Design review of the part built by this model. Coordinates are the model's own, in mm. A direction names the side the tool comes from. Round coordinates to 2 decimals unless told otherwise and drop trailing zeros. Order: outer loops, then holes, each group sorted by start corner. A loop starts at its lowest first (then second) coordinate and runs counter-clockwise, first axis right, second up. Notation, with made-up numbers: (66.5, 49.5) - (122.5, 49.5) arc R32 cw to (122.5, 82.5) - close; hole circle Ø8 at (77.5, 88.25). An arc over 180 degrees is marked (long way). Write item = value, one per line.
Autodesk Inventor part; units mm, degrees
ref_plane "YZ Plane" through (0, 0, 0) normal (1, 0, 0) x (0, 1, 0)
ref_plane "XZ Plane" through (0, 0, 0) normal (0, 1, 0) x (-1, 0, 0)
ref_plane "XY Plane" through (0, 0, 0) normal (0, 0, 1) x (1, 0, 0)
sketch "Esquisse1" plane through (0, 0, 0) normal (0, 1, 0) x (-1, 0, 0)
  line L0 (0, 0) -> (250, 0)
  line L1 (250, 0) -> (250, -32)
  line L2 (250, -32) -> (0, -32)
  line L3 (0, -32) -> (0, 0)
  circle A0 centre (2, -2) radius 1.5
  line L4 (250, -16) -> (0, -16) construction
  circle A1 centre (2, -30) radius 1.5
  circle A2 centre (51.1, -2) radius 1.5
  circle A3 centre (51.1, -30) radius 1.5
  circle A4 centre (100.2, -2) radius 1.5
  circle A5 centre (100.2, -30) radius 1.5
  circle A6 centre (149.3, -2) radius 1.5
  circle A7 centre (149.3, -30) radius 1.5
  circle A8 centre (198.4, -2) radius 1.5
  circle A9 centre (198.4, -30) radius 1.5
  circle A10 centre (247.5, -2) radius 1.5
  circle A11 centre (247.5, -30) radius 1.5
  dimension "d0" = 32
  dimension "d1" = 250
  dimension "d2" = 2
  dimension "d3" = 2
  dimension "d4" = 3
  dimension "d7" = 49.1
extrude "Extrusion1" add sketch "Esquisse1" along normal blind 1.6
sketch "Esquisse2" plane through (0, 1.6, 0) normal (0, 1, 0) x (1, 0, 0)
  circle A0 centre (-247.5, 30) radius 1.5 construction
  circle A1 centre (-247.5, 2) radius 1.5 construction
  circle A2 centre (-198.4, 30) radius 1.5 construction
  circle A3 centre (-198.4, 2) radius 1.5 construction
  circle A4 centre (-149.3, 30) radius 1.5 construction
  circle A5 centre (-149.3, 2) radius 1.5 construction
  circle A6 centre (-100.2, 30) radius 1.5 construction
  circle A7 centre (-100.2, 2) radius 1.5 construction
  circle A8 centre (-51.1, 30) radius 1.5 construction
  circle A9 centre (-51.1, 2) radius 1.5 construction
  circle A10 centre (-2, 30) radius 1.5 construction
  circle A11 centre (-2, 2) radius 1.5 construction
  line L0 (-250, 0) -> (0, 0) construction
  line L1 (0, 0) -> (0, 32) construction
  line L2 (0, 32) -> (-250, 32) construction
  line L3 (-250, 32) -> (-250, 0) construction
  line L4 (-246, 9.5) -> (-234, 9.5)
  line L5 (-234, 9.5) -> (-234, 21.5)
  line L6 (-234, 21.5) -> (-246, 21.5)
  line L7 (-246, 21.5) -> (-246, 9.5)
  dimension "d14" = 12
  dimension "d15" = 9.5
  dimension "d16" = 4
extrude "Extrusion2" add sketch "Esquisse2" along normal blind 7.7
sketch "Esquisse3" plane through (-246, 1.6, -21.5) normal (-1, 0, 0) x (0, 0, 1)
  circle A0 centre (4, 6) radius 1.1
  line L0 (-10.5, 0) -> (21.5, 0)
  line L1 (0, 0) -> (0, 7.7)
  line L2 (-10.5, -1.6) -> (21.5, -1.6)
  line L3 (5.5, -1.6) -> (5.5, 11.8569) construction
  dimension "d19" = 6
  dimension "d20" = 2.2
  dimension "d21" = 4
extrude "Extrusion3" add sketch "Esquisse3" along normal blind 7
sketch "Esquisse4" plane through (0, 1.6, 0) normal (0, 1, 0) x (1, 0, 0)
  line L0 (-246, 9.5) -> (-246, 21.5)
  line L1 (-246, 21.5) -> (-234, 21.5)
  line L2 (-234, 21.5) -> (-234, 9.5)
  line L3 (-234, 9.5) -> (-246, 9.5)
  circle A0 centre (-247.5, 30) radius 1.5
  circle A1 centre (-247.5, 2) radius 1.5
  circle A2 centre (-198.4, 30) radius 1.5
  circle A3 centre (-198.4, 2) radius 1.5
  circle A4 centre (-149.3, 30) radius 1.5
  circle A5 centre (-149.3, 2) radius 1.5
  circle A6 centre (-100.2, 30) radius 1.5
  circle A7 centre (-100.2, 2) radius 1.5
  circle A8 centre (-51.1, 30) radius 1.5
  circle A9 centre (-51.1, 2) radius 1.5
  circle A10 centre (-2, 30) radius 1.5
  circle A11 centre (-2, 2) radius 1.5
  line L4 (-250, 0) -> (0, 0)
  line L5 (0, 0) -> (0, 32)
  line L6 (0, 32) -> (-250, 32)
  line L7 (-250, 32) -> (-250, 0)
  line L8 (0, 0) -> (0, 32) construction
  line L9 (0, 16) -> (-250, 16) construction
  line L10 (-200, 19) -> (-190, 19)
  line L11 (-190, 19) -> (-190, 13)
  line L12 (-190, 13) -> (-200, 13)
  line L13 (-200, 13) -> (-200, 19)
  line L14 (-190, 16) -> (-200, 16) construction
  line L15 (-195, 19) -> (-195, 13) construction
  dimension "d24" = 10
  dimension "d26" = 6
  dimension "d29" = 55
extrude "Extrusion4" add sketch "Esquisse4" along normal blind 10 contours L10 L11 L12 L13
pattern_linear "Réseau rectangulaire1" count 7 spacing 22.1667 along (1, 0, 0) of "Extrusion4"
sketch "Esquisse6" plane through (0, 0, 0) normal (0, -1, 0) x (1, 0, 0)
  line L0 (-177.8333, -13) -> (-177.8333, -19)
  line L1 (-190, -19) -> (-190, -13)
  line L2 (-188.9167, -13) -> (-178.9167, -13)
  line L3 (-178.9167, -13) -> (-178.9167, -19)
  line L4 (-178.9167, -19) -> (-188.9167, -19)
  line L5 (-188.9167, -19) -> (-188.9167, -13)
  line L6 (-188.9167, -16) -> (-178.9167, -16) construction
  line L7 (-177.8333, -19) -> (-177.8333, -13) construction
  line L8 (-177.8333, -16) -> (-190, -16) construction
  line L9 (-190, -13) -> (-190, -19) construction
  point P0 (0, 0)
  point P1 (-183.9167, -16)
  dimension "d33" = 10
  dimension "d34" = 6
extrude "Extrusion5" add sketch "Esquisse6" along normal blind 10
sketch "Esquisse9" plane through (0, 0, 0) normal (0, -1, 0) x (1, 0, 0)
  line L0 (0, 0) -> (-250, 0)
  line L1 (-250, 0) -> (-250, -32)
  line L2 (-250, -32) -> (0, -32)
  line L3 (0, -32) -> (0, 0)
  circle A0 centre (-2, -2) radius 1.5
  circle A1 centre (-2, -30) radius 1.5
  circle A2 centre (-51.1, -2) radius 1.5
  circle A3 centre (-51.1, -30) radius 1.5
  circle A4 centre (-100.2, -30) radius 1.5
  circle A5 centre (-100.2, -2) radius 1.5
  circle A6 centre (-149.3, -2) radius 1.5
  circle A7 centre (-149.3, -30) radius 1.5
  circle A8 centre (-198.4, -2) radius 1.5
  circle A9 centre (-198.4, -30) radius 1.5
  circle A10 centre (-247.5, -2) radius 1.5
  circle A11 centre (-247.5, -30) radius 1.5
  line L4 (-178.9167, -13) -> (-178.9167, -19)
  line L5 (-178.9167, -19) -> (-188.9167, -19)
  line L6 (-188.9167, -19) -> (-188.9167, -13)
  line L7 (-188.9167, -13) -> (-178.9167, -13)
  line L8 (-178.9167, -13) -> (-178.9167, -19) construction
  line L9 (-178.9167, -16) -> (-142, -16) construction
  line L10 (-142, -1) -> (-142, -31) construction
  circle A12 centre (-173.9167, -22.5) radius 1.65
  circle A13 centre (-167.9167, -22.5) radius 1.65
  circle A14 centre (-161.9167, -22.5) radius 1.65
  circle A15 centre (-173.9167, -9.5) radius 1.65
  circle A16 centre (-167.9167, -9.5) radius 1.65
  circle A17 centre (-161.9167, -9.5) radius 1.65
  dimension "d51" = 6
  dimension "d56" = 3.3
  dimension "d57" = 13
  dimension "d58" = 5
extrude "Extrusion8" add sketch "Esquisse9" along normal blind 10 contours A12 | A13 | A14 | A15 | A16 | A17
sketch "Esquisse11" plane through (0, 1.6, 0) normal (0, 1, 0) x (1, 0, 0)
  line L0 (-57, 19) -> (-57, 13)
  line L1 (-57, 13) -> (-67, 13)
  line L2 (-67, 13) -> (-67, 19)
  line L3 (-67, 19) -> (-57, 19)
  line L4 (-79.1667, 19) -> (-79.1667, 13)
  line L5 (-79.1667, 13) -> (-89.1667, 13)
  line L6 (-89.1667, 13) -> (-89.1667, 19)
  line L7 (-89.1667, 19) -> (-79.1667, 19)
  line L8 (-101.3333, 19) -> (-101.3333, 13)
  line L9 (-101.3333, 13) -> (-111.3333, 13)
  line L10 (-111.3333, 13) -> (-111.3333, 19)
  line L11 (-111.3333, 19) -> (-101.3333, 19)
  line L12 (-123.5, 19) -> (-123.5, 13)
  line L13 (-123.5, 13) -> (-133.5, 13)
  line L14 (-133.5, 13) -> (-133.5, 19)
  line L15 (-133.5, 19) -> (-123.5, 19)
  line L16 (-145.6667, 19) -> (-145.6667, 13)
  line L17 (-145.6667, 13) -> (-155.6667, 13)
  line L18 (-155.6667, 13) -> (-155.6667, 19)
  line L19 (-155.6667, 19) -> (-145.6667, 19)
  line L20 (-167.8333, 19) -> (-167.8333, 13)
  line L21 (-167.8333, 13) -> (-177.8333, 13)
  line L22 (-177.8333, 13) -> (-177.8333, 19)
  line L23 (-177.8333, 19) -> (-167.8333, 19)
  line L24 (-190, 19) -> (-190, 13)
  line L25 (-190, 13) -> (-200, 13)
  line L26 (-200, 13) -> (-200, 19)
  line L27 (-200, 19) -> (-190, 19)
  line L28 (-246, 9.5) -> (-246, 21.5)
  line L29 (-246, 21.5) -> (-234, 21.5)
  line L30 (-234, 21.5) -> (-234, 9.5)
  line L31 (-234, 9.5) -> (-246, 9.5)
  circle A0 centre (-247.5, 30) radius 1.5
  circle A1 centre (-247.5, 2) radius 1.5
  circle A2 centre (-198.4, 30) radius 1.5
  circle A3 centre (-198.4, 2) radius 1.5
  circle A4 centre (-149.3, 30) radius 1.5
  circle A5 centre (-149.3, 2) radius 1.5
  circle A6 centre (-100.2, 30) radius 1.5
  circle A7 centre (-100.2, 2) radius 1.5
  circle A8 centre (-51.1, 30) radius 1.5
  circle A9 centre (-51.1, 2) radius 1.5
  circle A10 centre (-2, 30) radius 1.5
  circle A11 centre (-2, 2) radius 1.5
  line L32 (-250, 0) -> (0, 0)
  line L33 (0, 0) -> (0, 32)
  line L34 (0, 32) -> (-250, 32)
  line L35 (-250, 32) -> (-250, 0)
  line L36 (-52, 25) -> (0, 25)
  line L37 (0, 25) -> (0, 7)
  line L38 (0, 7) -> (-52, 7)
  line L39 (-52, 7) -> (-52, 25)
  line L40 (-52, 16) -> (0, 16) construction
  line L41 (0, 0) -> (0, 32) construction
  line L42 (0, 16) -> (-57, 16) construction
  line L43 (-57, 19) -> (-57, 13) construction
  dimension "d61" = 18
  dimension "d62" = 52
extrude "Extrusion9" add sketch "Esquisse11" along normal blind 4.5 contours L38 L39 L36 L33
sketch "Esquisse12" plane through (0, 6.1, 0) normal (0, 1, 0) x (1, 0, 0)
  line L0 (0, 25) -> (-52, 25)
  line L1 (-52, 25) -> (-52, 7)
  line L2 (-52, 7) -> (0, 7)
  line L3 (0, 7) -> (0, 25)
  line L4 (0, 32) -> (0, 0) construction
  line L5 (0, 16) -> (-52, 16) construction
  line L6 (-52, 25) -> (-52, 7) construction
  line L7 (-7.5, 12.25) -> (0, 12.25)
  line L8 (0, 12.25) -> (0, 19.75)
  line L9 (0, 19.75) -> (-7.5, 19.75)
  line L10 (-7.5, 19.75) -> (-7.5, 12.25)
  line L11 (0, 19.75) -> (1, 19.75)
  line L12 (1, 19.75) -> (1, 12.25)
  line L13 (1, 12.25) -> (0, 12.25)
  line L14 (0, 12.25) -> (0, 19.75)
  point P0 (0, 16)
  dimension "d65" = 7.5
  dimension "d66" = 7.5
  dimension "d69" = 1
extrude "Extrusion10" add sketch "Esquisse12" along normal blind 4 contours L11 L12 L13 L3 | L3 L7 L10 L9
sketch "Esquisse13" plane through (1, 6.1, -12.25) normal (1, 0, 0) x (0, 0, -1)
  line L0 (0, 0) -> (7.5, 0)
  line L1 (7.5, 0) -> (7.5, 4)
  line L2 (0, 4) -> (7.5, 4)
  line L3 (0, 0) -> (0, 4)
  line L4 (0.5, 3.5) -> (7, 3.5)
  line L5 (7, 3.5) -> (6.25, 0.5)
  line L6 (6.25, 0.5) -> (1.25, 0.5)
  line L7 (1.25, 0.5) -> (0.5, 3.5)
  line L8 (3.75, 3.5) -> (3.75, 0.5) construction
  line L9 (7.5, 4) -> (0, 4) construction
  line L10 (3.75, 4) -> (3.75, 0) construction
  line L11 (12.75, 0) -> (-5.25, 0) construction
  point P0 (-12.25, -6.1)
  dimension "d71" = 0.5
  dimension "d72" = 0.5
  dimension "d73" = 0.5
  dimension "d74" = 5
extrude "Extrusion11" cut sketch "Esquisse13" against normal blind 3 contours L4 L5 L6 L7
sketch "Esquisse14" plane through (0, 0, 0) normal (0, -1, 0) x (1, 0, 0)
  line L0 (0, -10) -> (-14, -10)
  line L1 (-14, -10) -> (-14, -22)
  line L2 (-14, -22) -> (0, -22)
  line L3 (0, -22) -> (0, -10)
  line L4 (0, -12.25) -> (0, -19.75) construction
  line L5 (0, -16) -> (-15.2374, -16) construction
  line L6 (0, -16) -> (-14, -16) construction
  line L7 (0, -32) -> (0, 0) construction
  line L8 (0.5, -22) -> (0, -22)
  line L9 (0, -22) -> (0, -10)
  line L10 (0, -10) -> (0.5, -10)
  line L11 (0.5, -10) -> (0.5, -22)
  dimension "d77" = 12
  dimension "d78" = 14
  dimension "d85" = 0.5
extrude "Extrusion12" add sketch "Esquisse14" along normal blind 6
sketch "Esquisse15" plane through (0, 0, -32) normal (1, 0, 0) x (0, 0, -1)
  line L0 (0, 0) -> (-10, 0)
  line L1 (0, 0) -> (0, 1.6)
  line L2 (-7, 1.6) -> (0, 1.6)
  line L3 (-7, 1.6) -> (-7, 6.1)
  line L4 (-12.25, 6.1) -> (-7, 6.1)
  line L5 (-19.75, 6.1) -> (-12.25, 6.1)
  line L6 (-25, 6.1) -> (-19.75, 6.1)
  line L7 (-25, 1.6) -> (-25, 6.1)
  line L8 (-32, 1.6) -> (-25, 1.6)
  line L9 (-32, 0) -> (-32, 1.6)
  line L10 (-22, -6) -> (-10, -6) construction
  line L11 (-16, -6) -> (-16, -0.2) construction
  circle A0 centre (-16, -3) radius 1.7
  line L12 (-10, 0) -> (-22, 0) construction
  line L13 (-22, 0) -> (-32, 0)
  line L14 (-10, 0) -> (-22, 0)
  dimension "d81" = 3
  dimension "d82" = 3.4
extrude "Extrusion13" cut sketch "Esquisse15" along normal mid plane 40 contours A0
sketch "Esquisse16" plane through (0, 0, 0) normal (0, -1, 0) x (1, 0, 0)
  line L0 (-142, 8) -> (-79, 8)
  line L1 (-79, 8) -> (-79, -40)
  line L2 (-79, -40) -> (-142, -40)
  line L3 (-142, -40) -> (-142, 8)
  line L4 (-79, -16) -> (-142, -16) construction
  line L5 (-250, 0) -> (-250, -32) construction
  line L6 (-250, -16) -> (0, -16) construction
  line L7 (0, -32) -> (0, -22) construction
  line L8 (-14, -10) -> (-14, -22) construction
  point P0 (0, 0)
  dimension "d86" = 63
  dimension "d87" = 48
  dimension "d91" = 108
extrude "Extrusion14" add sketch "Esquisse16" along normal blind 15
sketch "Esquisse17" plane through (0, 0, 0) normal (0, -1, 0) x (1, 0, 0)
  line L0 (-78, -26) -> (-68, -26)
  line L1 (-68, -26) -> (-68, -6)
  line L2 (-68, -6) -> (-78, -6)
  line L3 (-78, -6) -> (-78, -26)
  line L4 (-14, -22) -> (-14, -10) construction
  line L5 (-14, -16) -> (-79, -16) construction
  line L6 (-79, 0) -> (-79, -32) construction
  line L7 (-78, -16) -> (-68, -16) construction
  line L8 (0, -10) -> (0, 0) construction
  dimension "d92" = 68
  dimension "d93" = 10
  dimension "d94" = 20
extrude "Extrusion15" add sketch "Esquisse17" along normal blind 12
equation "\"d72\" = d71"
equation "\"d73\" = d71"
properties part number "electronics"
1) The part is to be moulded in two halves that separate along X. For faces 5 (the flat face through (-246, 5, -16)), 6 (the flat face through (-184, -5, -19)), 7 (the flat face through (-195, 7, -19)), 8 (the flat face through (-62, 7, -19)), say which applies: released by +X, released by -X, zero draft, split by the parting line, or undercut.
Findings:
face_5 = released by -X
face_6 = zero draft
face_7 = undercut
face_8 = undercut
2) Clearance check with flat-ended pins moving along their axes: pin 1 Ø6.5 at (y, z) = (6, -16) entering from +X; pin 2 Ø2 at (y, z) = (-5.5, -25) entering from +X; pin 3 Ø5 at (x, y) = (-126.5, 4.5) entering from +Z; pin 4 Ø8 at (x, y) = (-173, 8.5) entering from -Z. State where each tip first meets the part, or that it passes through.
Findings:
pin_1 = 1
pin_2 = -68
pin_3 = -13
pin_4 = -19
3) We need section B-B on z = -34.5. Write out the cut boundary in (x, y).
Findings:
outline = (-142, -15) - (-79, -15) - (-79, 0) - (-142, 0) - close
4) We need section C-C on x = -211.5. Write out the cut boundary in (y, z), and give its area (3 significant figures).
Findings:
outline = (0, -32) - (1.6, -32) - (1.6, 0) - (0, 0) - close
area = 51.2 mm^2
5) For faces 1 (the flat face through (-128, 7, -13)), 2 (the flat face through (0.5, -1.62, -17.25)), 3 (the flat face through (-240, 9.3, -16)), 4 (the flat face through (-234, 5, -15)), list the 3-axis set-ups (+Z, -Z, +X, -X, +Y, -Y) from which the entire face can be reached by the end or side of a thin tool; tool diameter is ignored.
Findings:
face_1 = +Z, +Y
face_2 = +Z, -Z, +X, -Y
face_3 = +Z, -Z, -X, +Y
face_4 = +Z, -Z, +Y
6) We need section A-A on x = -75. Write out the cut boundary in (y, z), and give its area (3 significant figures).
Findings:
outline = (-12, -26) - (0, -26) - (0, -32) - (1.6, -32) - (1.6, 0) - (0, 0) - (0, -6) - (-12, -6) - close
area = 291 mm^2
7) To check wall thickness, follow L1, parallel to Z at x = -100.2, y = 1.2; L2, parallel to X at y = -5, z = -12.5; L3, parallel to X at y = -7.5, z = -27. State the ranges of each line that lie inside material, in increasing order. Write a range as from..to.
Findings:
L1 = -32..-31.5, -28.5..-3.5, -0.5..0
L2 = -142..-79, -78..-68, -14..0.5
L3 = -142..-79
